The model under review builds one solid part; all positions refer to its coordinate system, in mm. Coordinates: 2 decimals unless noted, no trailing zeros. Order: outer loops, then holes, each group sorted by start corner. A loop starts at its lowest first (then second) coordinate and runs counter-clockwise, first axis right, second up. Notation, with made-up numbers: (31.25, 54) -> (38.25, 54) arc R6 cw to (38.25, 62) -> close; hole circle Ø11 at (-3.5, 63.5). An arc over 180 degrees is marked (long way). Use one line per item in the form item = value. Start each with the question number.
(1) Take a section at C-C (x = -327). State the section outline as (y, z) points, then the cut area to 3 significant figures.
(2) Take a section at B-B (y = -438). State the section outline as (x, z) points, then the cut area to 3 significant figures.
(3) Take a section at A-A (z = 856.5). State the section outline as (x, y) points, then the cut area to 3 significant figures.
(4) Wall thickness on line 1 along Z through (x, y) = (-6, -756.5): over which ranges is the line inside the solid? List them lowest first.
```python
from build123d import *

# Parameters (mm, degrees)
F0_W     = 800
F0_H     = 2225
F1_DEPTH = 800
F2_W     = 750
F2_H     = 2175
F3_DEPTH = 800
F4_W     = 750
F4_H     = 2175
F5_DEPTH = 800


with BuildPart() as f1:
    # F0 (on Front) → F1 (new body)
    with BuildSketch(Plane.XZ):
        Rectangle(F0_W, F0_H)
    extrude(amount=F1_DEPTH)

    # F2 (on face) → F3 (cut, through all)
    with BuildSketch(Plane.XZ.offset(800)):
        Rectangle(F2_W, F2_H)
    extrude(amount=-F3_DEPTH, mode=Mode.SUBTRACT)

    # F4 (on face) → F5 (cut, through all)
    with BuildSketch(Plane.YZ.offset(400)):
        with Locations((-400, 0)):
            Rectangle(F4_W, F4_H)
    extrude(amount=-F5_DEPTH, mode=Mode.SUBTRACT)


solid = f1.part
```
Findings:
q1.outline = (-800, -1112.5) -> (0, -1112.5) -> (0, -1087.5) -> (-800, -1087.5) -> close; (-800, 1087.5) -> (0, 1087.5) -> (0, 1112.5) -> (-800, 1112.5) -> close
q1.area = 40,000 mm²
q2.outline = (-400, -1112.5) -> (400, -1112.5) -> (400, -1087.5) -> (-400, -1087.5) -> close; (-400, 1087.5) -> (400, 1087.5) -> (400, 1112.5) -> (-400, 1112.5) -> close
q2.area = 40,000 mm²
q3.outline = (-400, -800) -> (-375, -800) -> (-375, -775) -> (-400, -775) -> close; (-400, -25) -> (-375, -25) -> (-375, 0) -> (-400, 0) -> close; (375, -800) -> (400, -800) -> (400, -775) -> (375, -775) -> close; (375, -25) -> (400, -25) -> (400, 0) -> (375, 0) -> close
q3.area = 2,500 mm²
q4.line_1 = -1112.5 to -1087.5, 1087.5 to 1112.5
